from build123d import *

# Parameters (mm, degrees)
SKETCH1_R                                           = 5
BOSS_EXTRUDE1_DEPTH                                 = 8
M4_CLEARANCE_HOLE1_D                                = 4.3
F_20_0MM_TRANSITIONAL_DOWEL_HOLE1_D                 = 21.5
CBORE_FOR_M4_HEX_SOCKET_HEAD_CAP_SCREW3_D           = 4.8
CBORE_FOR_M4_HEX_SOCKET_HEAD_CAP_SCREW3_CBORE_D     = 8
CBORE_FOR_M4_HEX_SOCKET_HEAD_CAP_SCREW3_CBORE_DEPTH = 4.4
SKETCH12_R                                          = 30
CUT_EXTRUDE1_DEPTH                                  = 2
FILLET1_R                                           = 0.5


with BuildPart() as part:
    # Sketch1 → Boss-Extrude1 (new body)
    with BuildSketch(Plane.XY):
        with BuildLine():
            Line((0, 0), (-80, 0))
            Line((-80, 0), (-80, 175))
            ThreePointArc((-80, 175), (-40, 215), (0, 175))
            Line((0, 175), (0, 0))
        make_face()
        with Locations((-40, 175)):
            Circle(SKETCH1_R, mode=Mode.SUBTRACT)
    extrude(amount=BOSS_EXTRUDE1_DEPTH)

    # M4 Clearance Hole1 (through all)
    with Locations(Plane.XY.offset(8)):
        with Locations((-66.5, 14), (-13.5, 14), (-13.5, 50), (-66.5, 50)):
            Hole(M4_CLEARANCE_HOLE1_D / 2)

    # Ø20.0mm Transitional Dowel Hole1 (through all)
    with Locations(Plane.XY.offset(8)):
        with Locations((-40, 175)):
            Hole(F_20_0MM_TRANSITIONAL_DOWEL_HOLE1_D / 2)

    # CBORE for M4 Hex Socket Head Cap Screw3 (through all)
    with Locations(Plane(origin=(0, 0, 0), x_dir=(1, 0, 0), z_dir=(0, 0, -1))):
        with Locations((-40, -200), (-15.000221056, -174.999778948), (-40.000442109, -150.000000004), (-65.000221052, -175.000221056)):
            CounterBoreHole(CBORE_FOR_M4_HEX_SOCKET_HEAD_CAP_SCREW3_D / 2, CBORE_FOR_M4_HEX_SOCKET_HEAD_CAP_SCREW3_CBORE_D / 2, CBORE_FOR_M4_HEX_SOCKET_HEAD_CAP_SCREW3_CBORE_DEPTH)

    # Sketch12 → Cut-Extrude1 (cut)
    with BuildSketch(Plane.XY.offset(8)):
        with Locations((-40, 175)):
            Circle(SKETCH12_R)
    extrude(amount=-CUT_EXTRUDE1_DEPTH, mode=Mode.SUBTRACT)

    # Fillet1
    fillet1_edges = [part.edges().sort_by_distance(p)[0] for p in [
        (-70, 175, 6),
    ]]
    fillet(fillet1_edges, radius=FILLET1_R)


solid = part.part
Work out the finished part from the listing and answer in its coordinate system (mm). A direction names the side the tool comes from. Give positions to 0.01 mm unless a question says otherwise; leave off trailing zeros. Order: outer loops, then holes, each group sorted by start corner. A loop starts at its lowest first (then second) coordinate and runs counter-clockwise, first axis right, second up. Notation, with made-up numbers: (-6.75, -24.5) - (37.25, -24.5) arc R17 cw to (37.25, -9.5) - close; hole circle Ø1 at (50, 50.5). An arc over 180 degrees is marked (long way). Answer as CSV lines item,"result". Start each with the question number.
Q1. The part is cut by section A-A (x = -40). Give the number of separate pieces and of enclosed holes in the cut face, then the cut area to 3 significant figures.
Q2. For faces 1 (the face through (-38, 202, 4.4)), 2 (the face through (-46.503, 145.713, 7.26)), 3 (the face through (0, 89, 4)), determine the directions among +Z, -Z, +X, -X, +Y, -Y from which every point of the face is accessible in a straight line to the end or side of a thin tool.
Q3. Given pin 1 Ø5.5 at (x, y) = (-13.5, 50) entering from -Z; pin 2 Ø6.5 at (x, y) = (-39.5, 149.5) entering from -Z; pin 3 Ø7.5 at (x, y) = (-65, 175) entering from +Z; pin 4 Ø4 at (x, z) = (-31.5, 2.5) entering from +Y, each flat-ended and moving along its own axis, determine where each tip first touches the part or whether it passes through.
Q4. The part is cut by section B-B (y = 14). Write down the section's boundary in (x, z), then the cut area to 3 significant figures.
Q5. Find the intervals of material crossed by L1, parallel to Y at x = -40, z = 4.85; L2, parallel to Y at x = -13.5, z = 4.75; L3, parallel to X at y = 49.5, z = 6.75, in increasing order. Write a range as [from, to].
Q6. The mould has two halves that part along Y. Classify faces 4 (the face through (-39, 85, 8)), 5 (the face through (-39, 0, 4)), 6 (the face through (-40.88, 214.99, 3.94)), 7 (the face through (-39.69, 197.62, 5.21)): +Y half, -Y half, draft (parallel to the pull), parting line (faces both ways), or undercut.
Check result:
1,separate pieces,"4"
1,enclosed holes,"0"
1,area,"1,390 mm²"
2,face 1,"-Z"
2,face 2,"+Z"
2,face 3,"+Z, -Z, +X, +Y, -Y"
3,pin 1,"stops at z = 0"
3,pin 2,"stops at z = 4.4"
3,pin 3,"stops at z = 6"
3,pin 4,"stops at y = 214.47"
4,outline,"(-80, 0) - (-68.65, 0) - (-68.65, 8) - (-80, 8) - close; (-64.35, 0) - (-15.65, 0) - (-15.65, 8) - (-64.35, 8) - close; (-11.35, 0) - (0, 0) - (0, 8) - (-11.35, 8) - close"
4,area,"571 mm²"
5,L1,"y = [0, 147.6], [152.4, 164.25], [185.75, 197.6], [202.4, 215]"
5,L2,"y = [0, 11.85], [16.15, 47.85], [52.15, 173.13], [176.87, 204.96]"
5,L3,"x = [-80, -68.59], [-64.41, -15.59], [-11.41, 0]"
6,face 4,"draft"
6,face 5,"-Y half"
6,face 6,"+Y half"
6,face 7,"undercut"
